from build123d import *

# Parameters (mm, degrees)
F0_R     = 3
F1_DEPTH = 5
F2_DEPTH = 2
F3_R     = 5
F4_R     = 5
F0_R_2   = 15
F5_DEPTH = 5
F6_DEPTH = 5
F7_DEPTH = 3


# Not quite as in the source:
# - a feature names something its author has since deleted; it is built from what else it names


with BuildPart() as f1:
    # F0 (on Top) → F1 (new body)
    with BuildSketch(Plane.XY):
        Polygon((55.3523313466, 115.8730502097), (-55.3523313466, 115.8730502097), (-61.1258340385, 115.8730502097), (-69.7860880763, 110.8730502097), (-72.6728394223, 105.8730502097), (-128.0251707689, 10), (-130.9119221148, 5), (-130.9119221148, -5), (-128.0251707689, -10), (-72.6728394223, -105.8730502097), (-69.7860880763, -110.8730502097), (-61.1258340385, -115.8730502097), (-55.3523313466, -115.8730502097), (55.3523313466, -115.8730502097), (61.1258340385, -115.8730502097), (69.7860880763, -110.8730502097), (72.6728394223, -105.8730502097), (128.0251707689, -10), (130.9119221148, -5), (130.9119221148, 5), (128.0251707689, 10), (72.6728394223, 105.8730502097), (69.7860880763, 110.8730502097), (61.1258340385, 115.8730502097), align=None)
        with Locations((-62.5692097115, -108.3730502097)):
            Circle(F0_R, mode=Mode.SUBTRACT)
        with Locations((62.5692097115, -108.3730502097)):
            Circle(F0_R, mode=Mode.SUBTRACT)
        with Locations((-125.1384194229, 0)):
            Circle(F0_R, mode=Mode.SUBTRACT)
        Polygon((-119.364916731, -5), (-119.364916731, 0), (-119.364916731, 5), (-64.0125853844, 100.8730502097), (-59.6824583655, 103.3730502097), (-55.3523313466, 105.8730502097), (55.3523313466, 105.8730502097), (59.6824583655, 103.3730502097), (64.0125853844, 100.8730502097), (119.364916731, 5), (119.364916731, 0), (119.364916731, -5), (64.0125853844, -100.8730502097), (59.6824583655, -103.3730502097), (55.3523313466, -105.8730502097), (-55.3523313466, -105.8730502097), (-59.6824583655, -103.3730502097), (-64.0125853844, -100.8730502097), align=None, mode=Mode.SUBTRACT)
        with Locations((-62.5692097115, 108.3730502097)):
            Circle(F0_R, mode=Mode.SUBTRACT)
        with Locations((125.1384194229, 0)):
            Circle(F0_R, mode=Mode.SUBTRACT)
        with Locations((62.5692097115, 108.3730502097)):
            Circle(F0_R, mode=Mode.SUBTRACT)
        with BuildLine():
            Line((-59.6824583655, 103.3730502097), (-64.0125853844, 100.8730502097))
            Line((-64.0125853844, 100.8730502097), (-14.0125853844, 14.2705098312))
            ThreePointArc((-14.0125853844, 14.2705098312), (-10, 17.3205080757), (-5.3523313466, 19.2705098312))
            Line((-5.3523313466, 19.2705098312), (-55.3523313466, 105.8730502097))
            Line((-55.3523313466, 105.8730502097), (-59.6824583655, 103.3730502097))
        make_face()
        with BuildLine():
            Line((55.3523313466, 105.8730502097), (5.3523313466, 19.2705098312))
            ThreePointArc((5.3523313466, 19.2705098312), (10, 17.3205080757), (14.0125853844, 14.2705098312))
            Line((14.0125853844, 14.2705098312), (64.0125853844, 100.8730502097))
            Line((64.0125853844, 100.8730502097), (59.6824583655, 103.3730502097))
            Line((59.6824583655, 103.3730502097), (55.3523313466, 105.8730502097))
        make_face()
        with BuildLine():
            Line((119.364916731, 5), (19.364916731, 5))
            ThreePointArc((19.364916731, 5), (19.8405939253, 2.5200858497), (20, 0))
            ThreePointArc((20, 0), (19.8405939253, -2.5200858497), (19.364916731, -5))
            Line((19.364916731, -5), (119.364916731, -5))
            Line((119.364916731, -5), (119.364916731, 0))
            Line((119.364916731, 0), (119.364916731, 5))
        make_face()
        with BuildLine():
            ThreePointArc((14.0125853844, -14.2705098312), (10, -17.3205080757), (5.3523313466, -19.2705098312))
            Line((5.3523313466, -19.2705098312), (55.3523313466, -105.8730502097))
            Line((55.3523313466, -105.8730502097), (59.6824583655, -103.3730502097))
            Line((59.6824583655, -103.3730502097), (64.0125853844, -100.8730502097))
            Line((64.0125853844, -100.8730502097), (14.0125853844, -14.2705098312))
        make_face()
        with BuildLine():
            Line((-14.0125853844, -14.2705098312), (-64.0125853844, -100.8730502097))
            Line((-64.0125853844, -100.8730502097), (-59.6824583655, -103.3730502097))
            Line((-59.6824583655, -103.3730502097), (-55.3523313466, -105.8730502097))
            Line((-55.3523313466, -105.8730502097), (-5.3523313466, -19.2705098312))
            ThreePointArc((-5.3523313466, -19.2705098312), (-10, -17.3205080757), (-14.0125853844, -14.2705098312))
        make_face()
        with BuildLine():
            Line((-119.364916731, 5), (-119.364916731, 0))
            Line((-119.364916731, 0), (-119.364916731, -5))
            Line((-119.364916731, -5), (-19.364916731, -5))
            ThreePointArc((-19.364916731, -5), (-20, 0), (-19.364916731, 5))
            Line((-19.364916731, 5), (-119.364916731, 5))
        make_face()
    extrude(amount=F1_DEPTH)

    # F0 (on Top) → F2 (join)
    with BuildSketch(Plane.XY):
        with Locations((-125.1384194229, 0)):
            Circle(F0_R)
        with Locations((-62.5692097115, 108.3730502097)):
            Circle(F0_R)
        with Locations((62.5692097115, 108.3730502097)):
            Circle(F0_R)
        with Locations((125.1384194229, 0)):
            Circle(F0_R)
        with Locations((62.5692097115, -108.3730502097)):
            Circle(F0_R)
        with Locations((-62.5692097115, -108.3730502097)):
            Circle(F0_R)
    extrude(amount=F2_DEPTH)

    # F3
    f3_edges = [f1.edges().sort_by_distance(p)[0] for p in [
        (-130.911922, 5, 2.5),
        (-130.911922, -5, 2.5),
        (-69.786088, -110.87305, 2.5),
        (-61.125834, -115.87305, 2.5),
        (61.125834, -115.87305, 2.5),
        (69.786088, -110.87305, 2.5),
        (130.911922, -5, 2.5),
        (130.911922, 5, 2.5),
        (69.786088, 110.87305, 2.5),
        (61.125834, 115.87305, 2.5),
        (-61.125834, 115.87305, 2.5),
        (-69.786088, 110.87305, 2.5),
    ]]
    fillet(f3_edges, radius=F3_R)

    # F4
    f4_edges = [f1.edges().sort_by_distance(p)[0] for p in [
        (-64.012585, 100.87305, 2.5),
        (-55.352331, 105.87305, 2.5),
        (55.352331, 105.87305, 2.5),
        (64.012585, 100.87305, 2.5),
        (119.364917, 5, 2.5),
        (119.364917, -5, 2.5),
        (64.012585, -100.87305, 2.5),
        (55.352331, -105.87305, 2.5),
        (-55.352331, -105.87305, 2.5),
        (-64.012585, -100.87305, 2.5),
        (-119.364917, -5, 2.5),
        (-119.364917, 5, 2.5),
    ]]
    fillet(f4_edges, radius=F4_R)

    # F0 (on Top) → F5 (join)
    with BuildSketch(Plane.XY):
        with BuildLine():
            ThreePointArc((-14.0125853844, 14.2705098312), (-17.3205080757, 10), (-19.364916731, 5))
            ThreePointArc((-19.364916731, 5), (-20, 0), (-19.364916731, -5))
            ThreePointArc((-19.364916731, -5), (-17.3205080757, -10), (-14.0125853844, -14.2705098312))
            ThreePointArc((-14.0125853844, -14.2705098312), (-10, -17.3205080757), (-5.3523313466, -19.2705098312))
            ThreePointArc((-5.3523313466, -19.2705098312), (0, -20), (5.3523313466, -19.2705098312))
            ThreePointArc((5.3523313466, -19.2705098312), (10, -17.3205080757), (14.0125853844, -14.2705098312))
            ThreePointArc((14.0125853844, -14.2705098312), (17.3205080757, -10), (19.364916731, -5))
            ThreePointArc((19.364916731, -5), (19.8405939253, -2.5200858497), (20, 0))
            ThreePointArc((20, 0), (19.8405939253, 2.5200858497), (19.364916731, 5))
            ThreePointArc((19.364916731, 5), (17.3205080757, 10), (14.0125853844, 14.2705098312))
            ThreePointArc((14.0125853844, 14.2705098312), (10, 17.3205080757), (5.3523313466, 19.2705098312))
            ThreePointArc((5.3523313466, 19.2705098312), (0, 20), (-5.3523313466, 19.2705098312))
            ThreePointArc((-5.3523313466, 19.2705098312), (-10, 17.3205080757), (-14.0125853844, 14.2705098312))
        make_face()
        Circle(F0_R_2, mode=Mode.SUBTRACT)
    extrude(amount=F5_DEPTH)

    # F0 (on Top) → F6 (join)
    with BuildSketch(Plane.XY):
        Circle(F0_R_2)
    extrude(amount=F6_DEPTH)

    # F0 (on Top) → F7 (cut)
    with BuildSketch(Plane.XY):
        Circle(F0_R_2)
    extrude(amount=F7_DEPTH, mode=Mode.SUBTRACT)


solid = f1.part
Input: part model. Units: mm. Frame: model coordinates. A direction names the side the tool comes from. Round coordinates to 2 decimals unless told otherwise and drop trailing zeros. Loops run counter-clockwise (first coordinate to the right, second up) from the corner with the lowest first, then second, coordinate; pieces in that order, holes last. Notation, with made-up numbers: M 7.5,1.25 L 47.5,1.25 A34 cw 47.5,33.25 Z; hole C 74,31.25 d3. An arc over 180 degrees is marked long. Answer as CSV lines item,"result". Start each with the question number.
(1) First-contact query: pin 1 (3 mm diameter, centred on x = -63, y = 107.5, fed in from +Z); pin 2 (9.5 mm diameter, centred on x = -62.57, y = 108.37, fed in from +Z); pin 3 (1.5 mm diameter, centred on x = 84, z = 2, fed in from +Y); pin 4 (1.5 mm diameter, centred on y = 43.5, z = 3, fed in from -X). Flat tips, straight axial feed; report the tip coordinate or a pass-through.
(2) Section D-D, the plane y = 0. Output: boundary loops of the cut face in (x, z).
(3) Reachability of faces 1 (the flat face through (125, 0, 2)), 2 (the flat face through (0, 0, 3)), 3 (the flat face through (92, -52.4, 2.5)) from +Z, -Z, +X, -X, +Y, -Y: full face, straight path, thin tool, end or side. Return the list, or none.
(4) Draft query along X for faces 4 (the flat face through (-1, 1, 5)), 5 (the flat face through (36.53, 53.27, 2.46)). Return one class per face: released by +X, released by -X, zero draft, split by the parting line, or undercut.
(5) Section C-C, the plane x = 31.5. Output: boundary loops of the cut face in (y, z).
(6) Line query: line 1 (Y direction, x = 0, z = 1.95); line 2 (Y direction, x = 36, z = 2.7); line 3 (Y direction, x = -113, z = 2.2). Output: solid intervals per line, ascending. Write a range as [from, to].
(7) Section A-A, the plane x = 0. Output: boundary loops of the cut face in (y, z), plus the area to 3 significant figures.
(8) Section B-B, the plane y = -78.5. Output: boundary loops of the cut face in (x, z).
Values found:
1,pin 1,"stops at z = 2"
1,pin 2,"stops at z = 5"
1,pin 3,"stops at y = 87.55"
1,pin 4,"stops at x = -109.12"
2,outline,"M -130.91,0 L -15,0 L -15,3 L 15,3 L 15,0 L 130.91,0 L 130.91,5 L 128.14,5 L 128.14,2 L 122.14,2 L 122.14,5 L -122.14,5 L -122.14,2 L -128.14,2 L -128.14,5 L -130.91,5 Z"
3,face 1,"+Z"
3,face 2,"-Z"
3,face 3,"+Z, -Z"
4,face 4,"zero draft"
4,face 5,"undercut"
5,outline,"M -115.87,0 L -105.87,0 L -105.87,5 L -115.87,5 Z; M -64.56,0 L -44.56,0 L -44.56,5 L -64.56,5 Z; M -5,0 L 5,0 L 5,5 L -5,5 Z; M 44.56,0 L 64.56,0 L 64.56,5 L 44.56,5 Z; M 105.87,0 L 115.87,0 L 115.87,5 L 105.87,5 Z"
6,line 1,"y = [-115.87, -105.87], [-20, -15], [15, 20], [105.87, 115.87]"
6,line 2,"y = [-115.87, -105.87], [-72.35, -52.35], [-5, 5], [52.35, 72.35], [105.87, 115.87]"
6,line 3,"y = [-36.02, -16.02], [-5.56, 5.56], [16.02, 36.02]"
7,outline,"M -115.87,0 L -105.87,0 L -105.87,5 L -115.87,5 Z; M -20,0 L -15,0 L -15,3 L 15,3 L 15,0 L 20,0 L 20,5 L -20,5 Z; M 105.87,0 L 115.87,0 L 115.87,5 L 105.87,5 Z"
7,area,"210 mm²"
8,outline,"M -88.48,0 L -76.93,0 L -76.93,5 L -88.48,5 Z; M -51.1,0 L -39.55,0 L -39.55,5 L -51.1,5 Z; M 39.55,0 L 51.1,0 L 51.1,5 L 39.55,5 Z; M 76.93,0 L 88.48,0 L 88.48,5 L 76.93,5 Z"
